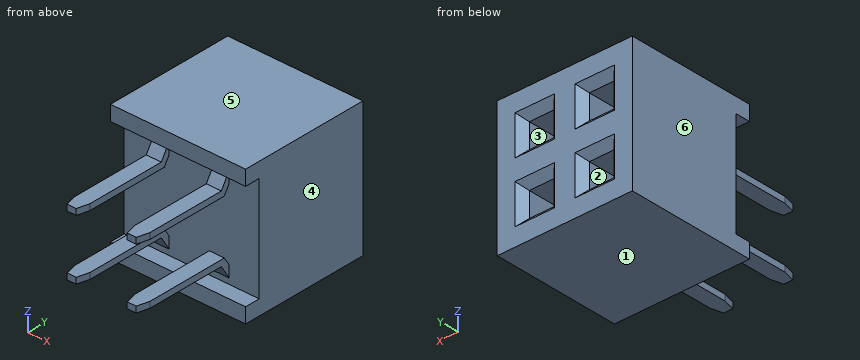
from build123d import *

# Parameters (mm, degrees)
EXTRUDE_1_DEPTH            = 1
SKETCH_3_W                 = 0.814720046
SKETCH_3_H                 = 0.814720046
CUT_EXTRUDE_1_DEPTH        = 3.5
CHAMFER_1_SIZE             = 0.25
CHAMFER_1_OF_MIRROR_1_SIZE = 0.25
EXTRUDE_2_DEPTH            = 0.25
CHAMFER_2_SIZE             = 0.1
CHAMFER_2_SIZE2            = 0.4
CUT_EXTRUDE_2_DEPTH        = 8.514818694
EXTRUDE_4_DEPTH            = 0.25


with BuildPart() as part:
    # 草图1 → 凸台-拉伸1 (new, symmetric)
    with BuildSketch(Plane(origin=(0, 0, 0), x_dir=(0, 0, -1), z_dir=(1, 0, 0))):
        Polygon((-2.25, 0), (2.25, 0), (2.25, -4.3), (1.75, -4.3), (1.75, -3.8), (-1.75, -3.8), (-1.75, -4.3), (-2.25, -4.3), align=None)
    extrude(amount=EXTRUDE_1_DEPTH, both=True)

    # 草图3 → 切除-拉伸1 (cut)
    with BuildSketch(Plane(origin=(0, 0, 0), x_dir=(1, 0, 0), z_dir=(0, 1, 0))):
        with Locations((0, 1)):
            Rectangle(SKETCH_3_W, SKETCH_3_H)
    cut_extrude_1 = extrude(amount=-CUT_EXTRUDE_1_DEPTH, mode=Mode.SUBTRACT)

    # 倒角1
    chamfer_1_edges = [part.edges().sort_by_distance(p)[0] for p in [
        (-0.407360023, 0, -1),
        (0, 0, -0.592639977),
        (0.407360023, 0, -1),
        (0, 0, -1.407360023),
    ]]
    chamfer(chamfer_1_edges, length=CHAMFER_1_SIZE)

    # 镜向1: 切除-拉伸1 across plane
    add(cut_extrude_1.mirror(Plane.XY), mode=Mode.SUBTRACT)

    # 倒角1 of 镜向1
    chamfer_1_of_mirror_1_edges = [part.edges().sort_by_distance(p)[0] for p in [
        (-0.407360023, 0, 1),
        (0, 0, 0.592639977),
        (0.407360023, 0, 1),
        (0, 0, 1.407360023),
    ]]
    chamfer(chamfer_1_of_mirror_1_edges, length=CHAMFER_1_OF_MIRROR_1_SIZE)

    # 草图4 → 凸台-拉伸2 (add)
    with BuildSketch(Plane(origin=(0, 0, 0), x_dir=(0, 0, -1), z_dir=(1, 0, 0))):
        Polygon((1.562968954, -3.8), (1.1, -4.088782437), (1.1, -7.1), (0.9, -7.1), (0.9, -3.977816442), (1.18507098, -3.8), align=None)
    extrude(amount=EXTRUDE_2_DEPTH)

    # 倒角2
    chamfer_2_edges = [part.edges().sort_by_distance(p)[0] for p in [
        (0.25, -7.1, -1),
    ]]
    chamfer_2_side = [part.faces().sort_by_distance(p)[0] for p in [
        (0.125, -7.1, -1),
    ]]
    chamfer(chamfer_2_edges, length=CHAMFER_2_SIZE, length2=CHAMFER_2_SIZE2, reference=chamfer_2_side[0])

    # 草图5 → 切除-拉伸2 (cut, through all)
    with BuildSketch(Plane(origin=(0, 0, 0), x_dir=(1, 0, 0), z_dir=(0, 1, 0))):
        Polygon((0, 2.25), (-1, 2.25), (-1, -2.25), (1, -2.25), (1, 0), (0, 0), align=None)
    extrude(amount=-CUT_EXTRUDE_2_DEPTH, mode=Mode.SUBTRACT)

    # 镜向3: part across plane


with BuildPart() as part_1:
    add(part.part)
    add(part.part.mirror(Plane(origin=(0, 0, 0), x_dir=(0, 0, 1), z_dir=(1, 0, 0))))

    # 镜向4: part across plane


with BuildPart() as part_2:
    add(part_1.part)
    add(part_1.part.mirror(Plane(origin=(0, -7.1, 0), x_dir=(1, 0, 0), z_dir=(0, 0, -1))))

    # 草图6 → 凸台-拉伸4 (add)
    with BuildSketch(Plane(origin=(1, 0, 0), x_dir=(0, 0, -1), z_dir=(1, 0, 0))):
        Polygon((2.25, 0), (-2.25, 0), (-2.25, -4.3), (-1.75, -4.3), (-1.75, -3.8), (1.75, -3.8), (1.75, -4.3), (2.25, -4.3), align=None)
    extrude(amount=EXTRUDE_4_DEPTH)

    # 镜向5: part across face


with BuildPart() as part_3:
    add(part_2.part)
    add(part_2.part.mirror(Plane(origin=(-1, -1.961079545, 0), x_dir=(0, 0, 1), z_dir=(-1, 0, 0))))


solid = part_3.part
Part model, mm, in its own coordinate system. Face numbers are marked on the shaded views. A direction names the side the tool comes from. Round coordinates to 2 decimals unless told otherwise and drop trailing zeros. Write each loop counter-clockwise with the first axis right and the second up, starting at its lowest first coordinate (ties: lowest second). Pieces come first, ordered by that corner, then holes. Notation, with made-up numbers: M 40.25,8.5 L 76.25,8.5 A23 ccw 76.25,33.5 Z; hole C -3,40 d8. An arc over 180 degrees is marked long. Return JSON: item names as keys, results as strings. Group by question number.
(1) Saw through at C-C on z = -1. Write the cut outline in (x, y), then the cut area to 3 significant figures.
(2) Drill centre lines: probe 1 along X at (y, z) = (-3.25, 1.1); probe 2 along Z at (x, y) = (-0.2, -2); probe 3 along X at (y, z) = (-6.5, -1). Where is each one in solid material? Low to high.
(3) Pin check, flat tips, straight feed: pin 1 Ø0.7 at (x, z) = (0, 1) entering from +Y; pin 2 Ø0.7 at (y, z) = (-5, -1.5) entering from +X; pin 3 Ø0.5 at (y, z) = (-5.5, -1) entering from +X. Stop position of each tip, or through.
(4) Saw through at A-A on y = -5.5. Write the cut outline in (x, z), then the cut area to 3 significant figures.
(5) Two-plate mould, pull along X, no slides. Class the marked faces 3, 4, 5 and 6: +X half, -X half, draft (parallel to the pull), parting line (faces both ways), or undercut.
(6) Which spindle directions (+Z, -Z, +X, -X, +Y, -Y) get a long thin tool onto all of the face, cutting with end or side? Do the marked faces 1 and 2. Say none if no direction does.
(7) Saw through at D-D on y = -1.5. Write the cut outline in (x, z).
Returned:
{
 "1": {"outline": "M -3.25,-3.8 L 1.25,-3.8 L 1.25,0 L 0.66,0 L 0.41,-0.25 L 0.41,-3.5 L -0.41,-3.5 L -0.41,-0.25 L -0.66,0 L -1.34,0 L -1.59,-0.25 L -1.59,-3.5 L -2.41,-3.5 L -2.41,-0.25 L -2.66,0 L -3.25,0 Z; M -2.25,-6.7 L -2.15,-7.1 L -1.85,-7.1 L -1.75,-6.7 L -1.75,-3.92 L -2.25,-3.92 Z; M -0.25,-6.7 L -0.15,-7.1 L 0.15,-7.1 L 0.25,-6.7 L 0.25,-3.92 L -0.25,-3.92 Z", "area": "14.4 mm²"},
 "2": {"probe 1": "-3.25 to -2.41, -1.59 to -0.41, 0.41 to 1.25", "probe 2": "-2.25 to -1.41, -0.59 to 0.59, 1.41 to 2.25", "probe 3": "-2.25 to -1.75, -0.25 to 0.25"},
 "3": {"pin 1": "y = -3.5", "pin 2": "through", "pin 3": "x = 0.25"},
 "4": {"outline": "M -2.25,-1.1 L -1.75,-1.1 L -1.75,-0.9 L -2.25,-0.9 Z; M -2.25,0.9 L -1.75,0.9 L -1.75,1.1 L -2.25,1.1 Z; M -0.25,-1.1 L 0.25,-1.1 L 0.25,-0.9 L -0.25,-0.9 Z; M -0.25,0.9 L 0.25,0.9 L 0.25,1.1 L -0.25,1.1 Z", "area": "0.400 mm²"},
 "5": {"face 3": "undercut", "face 4": "+X half", "face 5": "draft", "face 6": "-X half"},
 "6": {"face 1": "-Z, +X, -X, +Y, -Y", "face 2": "+Y"},
 "7": {"outline": "M -3.25,-2.25 L 1.25,-2.25 L 1.25,2.25 L -3.25,2.25 Z; hole M -2.41,-1.41 L -1.59,-1.41 L -1.59,-0.59 L -2.41,-0.59 Z; hole M -2.41,0.59 L -1.59,0.59 L -1.59,1.41 L -2.41,1.41 Z; hole M -0.41,-1.41 L 0.41,-1.41 L 0.41,-0.59 L -0.41,-0.59 Z; hole M -0.41,0.59 L 0.41,0.59 L 0.41,1.41 L -0.41,1.41 Z"}
}
